from build123d import *

# Parameters (mm, degrees)
SKETCH1_W                                 = 246.825
SKETCH1_H                                 = 63.5
BOSS_EXTRUDE1_DEPTH                       = 17.5
HOLE1_AT_2_COUNT                          = 2
HOLE1_AT_2_PITCH                          = 44.45
HOLE1_AT_3_COUNT                          = 2
HOLE1_AT_3_PITCH                          = 165.1
HOLE1_AT_4_COUNT                          = 2
HOLE1_AT_4_PITCH                          = 170.978982627
F_4_CLEARANCE_HOLE1_AT_2_COUNT            = 2
F_4_CLEARANCE_HOLE1_AT_2_PITCH            = 74.93
F_4_CLEARANCE_HOLE1_AT_3_COUNT            = 2
F_4_CLEARANCE_HOLE1_AT_3_PITCH            = 135.89
F_4_CLEARANCE_HOLE1_AT_4_COUNT            = 2
F_4_CLEARANCE_HOLE1_AT_4_PITCH            = 50.8
F_4_CLEARANCE_HOLE1_AT_5_COUNT            = 2
F_4_CLEARANCE_HOLE1_AT_5_PITCH            = 90.527039607
F_4_CLEARANCE_HOLE1_AT_6_COUNT            = 2
F_4_CLEARANCE_HOLE1_AT_6_PITCH            = 145.074918921
F_21_64_0_32813_DIAMETER_HOLE1_AT_2_COUNT = 2
F_21_64_0_32813_DIAMETER_HOLE1_AT_2_PITCH = 119.253


with BuildPart() as part:
    # Sketch1 → Boss-Extrude1 (new body)
    with BuildSketch(Plane(origin=(0, 0, 0), x_dir=(1, 0, 0), z_dir=(0, 1, 0))):
        with Locations((28.1625, 0)):
            Rectangle(SKETCH1_W, SKETCH1_H)
    extrude(amount=BOSS_EXTRUDE1_DEPTH)

    # Sketch2 → Hole1 (revolve, cut)
    with BuildSketch(Plane(origin=(82.55, 0, 22.225), x_dir=(0, 0, -1), z_dir=(1, 0, 0))):
        Polygon((0, 0), (0, 17.5), (2.38125, 17.5), (2.38125, 5.02895), (2.75, 4.6602), (4.1275, 4.6602), (4.1275, 0.6225), (4.75, 0), align=None)
    hole1 = revolve(axis=Axis((82.55, -6.35, 22.225), (0, 1, 0)), mode=Mode.SUBTRACT)

    # Hole1 at 2: Hole1 ×2
    with Locations(*[(0, 0, -i * HOLE1_AT_2_PITCH) for i in range(1, HOLE1_AT_2_COUNT)]):
        add(hole1, mode=Mode.SUBTRACT)

    # Hole1 at 3: Hole1 ×2
    with Locations(*[(-i * HOLE1_AT_3_PITCH, 0, 0) for i in range(1, HOLE1_AT_3_COUNT)]):
        add(hole1, mode=Mode.SUBTRACT)

    # Hole1 at 4: Hole1 ×2
    with Locations(*[Vector(-0.9656157585206697, 0, -0.2599734734478725) * (i * HOLE1_AT_4_PITCH) for i in range(1, HOLE1_AT_4_COUNT)]):
        add(hole1, mode=Mode.SUBTRACT)

    # Sketch4 → #4 Clearance Hole1 (revolve, cut)
    with BuildSketch(Plane(origin=(-68.58, 0, -25.4), x_dir=(0, 0, -1), z_dir=(1, 0, 0))):
        Polygon((0, 0), (0, 17.5), (1.905, 17.5), (1.4732, 17.0682), (1.4732, 2.9718), (1.905, 2.54), (3.175, 2.54), (3.175, 0.254), (3.429, 0), align=None)
    f_4_clearance_hole1 = revolve(axis=Axis((-68.58, -6.35, -25.4), (0, 1, 0)), mode=Mode.SUBTRACT)

    # #4 Clearance Hole1 at 2: #4 Clearance Hole1 ×2
    with Locations(*[(i * F_4_CLEARANCE_HOLE1_AT_2_PITCH, 0, 0) for i in range(1, F_4_CLEARANCE_HOLE1_AT_2_COUNT)]):
        add(f_4_clearance_hole1, mode=Mode.SUBTRACT)

    # #4 Clearance Hole1 at 3: #4 Clearance Hole1 ×2
    with Locations(*[(i * F_4_CLEARANCE_HOLE1_AT_3_PITCH, 0, 0) for i in range(1, F_4_CLEARANCE_HOLE1_AT_3_COUNT)]):
        add(f_4_clearance_hole1, mode=Mode.SUBTRACT)

    # #4 Clearance Hole1 at 4: #4 Clearance Hole1 ×2
    with Locations(*[(0, 0, i * F_4_CLEARANCE_HOLE1_AT_4_PITCH) for i in range(1, F_4_CLEARANCE_HOLE1_AT_4_COUNT)]):
        add(f_4_clearance_hole1, mode=Mode.SUBTRACT)

    # #4 Clearance Hole1 at 5: #4 Clearance Hole1 ×2
    with Locations(*[Vector(0.8277084982047687, 0, 0.56115830386764) * (i * F_4_CLEARANCE_HOLE1_AT_5_PITCH) for i in range(1, F_4_CLEARANCE_HOLE1_AT_5_COUNT)]):
        add(f_4_clearance_hole1, mode=Mode.SUBTRACT)

    # #4 Clearance Hole1 at 6: #4 Clearance Hole1 ×2
    with Locations(*[Vector(0.9366884435330111, 0, 0.35016390412449033) * (i * F_4_CLEARANCE_HOLE1_AT_6_PITCH) for i in range(1, F_4_CLEARANCE_HOLE1_AT_6_COUNT)]):
        add(f_4_clearance_hole1, mode=Mode.SUBTRACT)

    # Sketch8 → 21/64 (0.32813) Diameter Hole1 (revolve, cut)
    with BuildSketch(Plane(origin=(-69.85, 0, 0), x_dir=(0, 0, -1), z_dir=(1, 0, 0))):
        Polygon((0, 0), (0, 17.5), (4.802251, 17.5), (4.167251, 16.865), (4.167251, 0.635), (4.802251, 0), align=None)
    f_21_64_0_32813_diameter_hole1 = revolve(axis=Axis((-69.85, -6.35, 0), (0, 1, 0)), mode=Mode.SUBTRACT)

    # 21/64 (0.32813) Diameter Hole1 at 2: 21/64 (0.32813) Diameter Hole1 ×2
    with Locations(*[(i * F_21_64_0_32813_DIAMETER_HOLE1_AT_2_PITCH, 0, 0) for i in range(1, F_21_64_0_32813_DIAMETER_HOLE1_AT_2_COUNT)]):
        add(f_21_64_0_32813_diameter_hole1, mode=Mode.SUBTRACT)


solid = part.part
Input: part model. Units: mm. Frame: model coordinates. A direction names the side the tool comes from. Coordinates: 2 decimals unless noted, no trailing zeros.
Q1. Draft query along Z for faces 1 (the face through (-95.25, 9, 0)), 2 (the face through (-78.52, 2.61, -21.33)), 3 (the face through (-71.257, 1.381, -27.107)). Return one class per face: +Z half, -Z half, draft (parallel to the pull), parting line (faces both ways), or undercut.
Q2. Contact query for flat-ended pins moving along their axis: pin 1 (5 mm diameter, centred on x = 82.55, z = 22.225, fed in from -Y); pin 2 (9.5 mm diameter, centred on x = 49.403, z = 0, fed in from +Y); pin 3 (7.5 mm diameter, centred on x = -82.55, z = 22.225, fed in from -Y). Output: stop coordinate, or through.
Q3. Material intervals for line 1 (Z direction, x = 67.31, y = 13.75); line 2 (Z direction, x = 67.31, y = 1.65) (3 decimals); line 3 (X direction, y = 13.5, z = 25.4) (3 decimals), sorted ascending.
Q4. Set-up query: faces 4 (the face through (69, 2.54, 27)), 5 (the face through (-80.437, 11.177, -23.324)). Return all of +Z, -Z, +X, -X, +Y, -Y with unobstructed straight access to the full face (end or side cutting, diameter ignored); none if empty.
Q5. Cut plane A-A (x = -82.55). Give the number of separate pieces and of enclosed holes in the cut face, then the cut area to 3 significant figures.
Working result:
1. face 1: draft
1. face 2: undercut
1. face 3: undercut
2. pin 1: stops at y = 4.91
2. pin 2: stops at y = 17.45
2. pin 3: stops at y = 4.66
3. line 1: z = -31.75 to -26.87, -23.93 to 23.93, 26.87 to 31.75
3. line 2: z = -31.75 to -28.575, -22.225 to 22.225, 28.575 to 31.75
3. line 3: x = -95.25 to -70.053, -67.107 to 4.877, 7.823 to 65.837, 68.783 to 151.575
4. face 4: -Y
4. face 5: +Y, -Y
5. separate pieces: 3
5. enclosed holes: 0
5. area: 911 mm2
